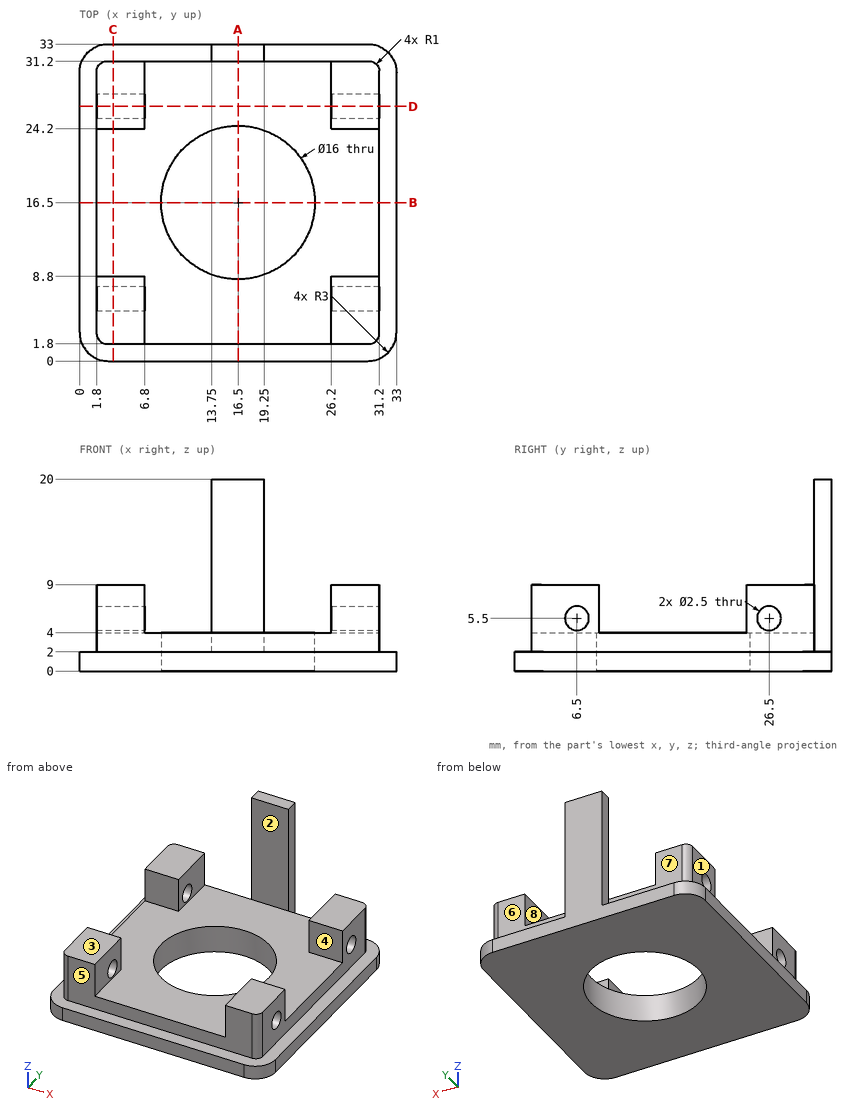
Source: three-view drawing plus pictorial views. Frame: mm from the lowest corner of the part. A direction names the side the tool comes from. Round coordinates to 2 decimals unless told otherwise and drop trailing zeros. Loops run counter-clockwise (first coordinate to the right, second up) from the corner with the lowest first, then second, coordinate; pieces in that order, holes last. Notation, with made-up numbers: M 60,62.25 L 100,62.25 A19 ccw 100,89.25 Z; hole C 9,24.25 d6. An arc over 180 degrees is marked long. Put each result on its own line as item: value. Start each with the question number.
(1) Section query D-D (y = 26.5). Return loops of the section in (x, z).
(2) Draft query along X for the marked faces 1, 2 and 3. Return one class per face: +X half, -X half, draft (parallel to the pull), parting line (faces both ways), or undercut.
(3) Material intervals for line 1 along Z through (x, y) = (3.7, 26.5); line 2 along Y through (x, z) = (2, 6.25); line 3 along X through (y, z) = (16.5, 2.55), sorted ascending. Write a range as [from, to].
(4) Contact query for flat-ended pins moving along their axis: pin 1 Ø3 at (y, z) = (26.5, 5.5) entering from +X; pin 2 Ø7.5 at (y, z) = (14, 7) entering from -X; pin 3 Ø4 at (x, y) = (28, 27.5) entering from +Z. Output: stop coordinate, or through.
(5) Section query A-A (x = 16.5). Return loops of the section in (y, z), then the cut area to 3 significant figures.
(6) Section query C-C (x = 3.5). Return loops of the section in (y, z), then the cut area to 3 significant figures.
(7) Section query B-B (y = 16.5). Return loops of the section in (x, z), then the cut area to 3 significant figures.
(8) Set-up query: the marked faces 4, 5, 6, 7 and 8. Return all of +Z, -Z, +X, -X, +Y, -Y with unobstructed straight access to the full face (end or side cutting, diameter ignored); none if empty.
Findings below:
1. outline: M 0,0 L 33,0 L 33,2 L 31.2,2 L 31.2,4.25 L 26.2,4.25 L 26.2,4 L 6.8,4 L 6.8,4.25 L 1.8,4.25 L 1.8,2 L 0,2 Z; M 1.8,6.75 L 6.8,6.75 L 6.8,9 L 1.8,9 Z; M 26.2,6.75 L 31.2,6.75 L 31.2,9 L 26.2,9 Z
2. face 1: -X half
2. face 2: undercut
2. face 3: draft
3. line 1: z = [0, 4.25], [6.75, 9]
3. line 2: y = [2.2, 5.5], [7.5, 8.8], [24.2, 25.5], [27.5, 30.8]
3. line 3: x = [1.8, 8.5], [24.5, 31.2]
4. pin 1: stops at x = 31.2
4. pin 2: stops at x = 1.8
4. pin 3: stops at z = 9
5. outline: M 0,0 L 8.5,0 L 8.5,4 L 1.8,4 L 1.8,2 L 0,2 Z; M 24.5,0 L 33,0 L 33,20 L 31.2,20 L 31.2,4 L 24.5,4 Z
5. area: 93.2 mm2
6. outline: M 0,0 L 33,0 L 33,2 L 31.2,2 L 31.2,9 L 24.2,9 L 24.2,4 L 8.8,4 L 8.8,9 L 1.8,9 L 1.8,2 L 0,2 Z; hole C 6.5,5.5 d2.5; hole C 26.5,5.5 d2.5
6. area: 185 mm2
7. outline: M 0,0 L 8.5,0 L 8.5,4 L 1.8,4 L 1.8,2 L 0,2 Z; M 24.5,0 L 33,0 L 33,2 L 31.2,2 L 31.2,4 L 24.5,4 Z
7. area: 60.8 mm2
8. face 4: +Z, +X, -X
8. face 5: +Z, +X, -X, -Y
8. face 6: +Z, +X, +Y
8. face 7: +Z, -X, +Y
8. face 8: +Z, +Y, -Y
